from build123d import *

# Parameters (mm, degrees)
SKETCH3_R           = 12.7
BOSS_EXTRUDE1_DEPTH = 381
SKETCH4_W           = 50.8
SKETCH4_H           = 50.8
BOSS_EXTRUDE2_DEPTH = 25.4
SKETCH5_W           = 50.8
SKETCH5_H           = 50.8
BOSS_EXTRUDE3_DEPTH = 25.4


with BuildPart() as part:
    # Sketch3 → Boss-Extrude1 (new body)
    with BuildSketch(Plane.XY):
        Circle(SKETCH3_R)
    extrude(amount=BOSS_EXTRUDE1_DEPTH)

    # Sketch4 → Boss-Extrude2 (add, symmetric)
    with BuildSketch(Plane(origin=(0, 0, 0), x_dir=(-1, 0, 0), z_dir=(0, 0, -1))):
        Rectangle(SKETCH4_W, SKETCH4_H)
    extrude(amount=BOSS_EXTRUDE2_DEPTH, both=True)

    # Sketch5 → Boss-Extrude3 (add, symmetric)
    with BuildSketch(Plane.XY.offset(381)):
        Rectangle(SKETCH5_W, SKETCH5_H)
    extrude(amount=BOSS_EXTRUDE3_DEPTH, both=True)


solid = part.part
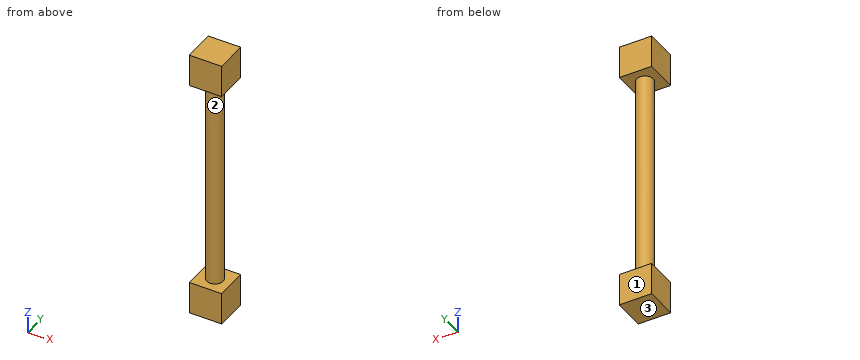
Input: part model. Units: mm. Frame: model coordinates. Face numbers are marked on the shaded views. Coordinates: 2 decimals unless noted, no trailing zeros. Loops run counter-clockwise (first coordinate to the right, second up) from the corner with the lowest first, then second, coordinate; pieces in that order, holes last.
Q1. Cut plane D-D (z = 242.5). Output: boundary loops of the cut face in (x, y).
Q2. Material intervals for line 1 (Z direction, x = -11, y = 8); line 2 (Y direction, x = -0.5, z = 92); line 3 (Y direction, x = -6.5, z = 146), sorted ascending.
Q3. Contact query for flat-ended pins moving along their axis: pin 1 (1 mm diameter, centred on y = 6.5, z = 110, fed in from +X); pin 2 (5 mm diameter, centred on y = -17, z = 63.5, fed in from +X); pin 3 (4 mm diameter, centred on x = -11.5, z = 103.5, fed in from +Y); pin 4 (1 mm diameter, centred on x = 9, z = 27.5, fed in from +Y). Output: stop coordinate, or through.
Q4. Cut plane A-A (x = -19). Output: boundary loops of the cut face in (y, z).
Q5. Draft query along Z for the marked faces 1, 2 and 3. Return one class per face: +Z half, -Z half, draft (parallel to the pull), parting line (faces both ways), or undercut.
Q6. Cut plane B-B (y = 0). Output: boundary loops of the cut face in (x, z), then the cut area to 3 significant figures.
Working result:
1. outline: circle Ø25.4 at (0, 0)
2. line 1: z = -25.4 to 25.4, 355.6 to 406.4
2. line 2: y = -12.69 to 12.69
2. line 3: y = -10.91 to 10.91
3. pin 1: stops at x = 11.19
3. pin 2: passes through
3. pin 3: stops at y = 8.43
3. pin 4: stops at y = 9.44
4. outline: (-25.4, -25.4) - (25.4, -25.4) - (25.4, 25.4) - (-25.4, 25.4) - close; (-25.4, 355.6) - (25.4, 355.6) - (25.4, 406.4) - (-25.4, 406.4) - close
5. face 1: draft
5. face 2: undercut
5. face 3: -Z half
6. outline: (-25.4, -25.4) - (25.4, -25.4) - (25.4, 25.4) - (12.7, 25.4) - (12.7, 355.6) - (25.4, 355.6) - (25.4, 406.4) - (-25.4, 406.4) - (-25.4, 355.6) - (-12.7, 355.6) - (-12.7, 25.4) - (-25.4, 25.4) - close
6. area: 13,500 mm2
